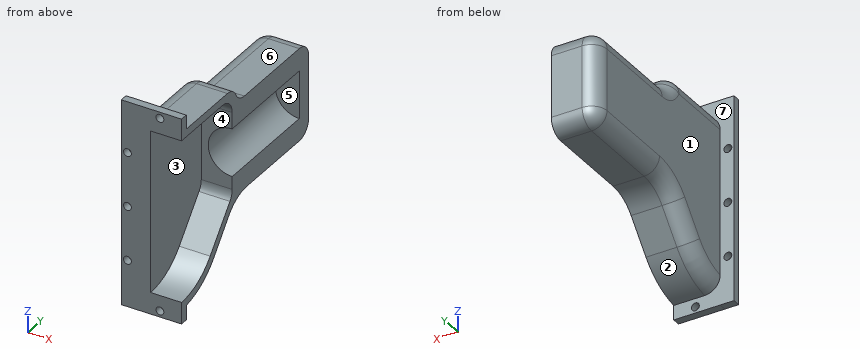
```python
from build123d import *

# Parameters (mm, degrees)
BOSS_EXTRUDE1_DEPTH   = 120
FILLET1_R             = 20
FILLET2_R             = 20
SKETCH2_W             = 18
SKETCH2_H             = 103
BOSS_EXTRUDE2_DEPTH   = 10
F_1_0MM_DOWEL_HOLE1_D = 10.2
F_1_0MM_DOWEL_HOLE2_D = 10.2
SKETCH7_R             = 31
CUT_EXTRUDE1_DEPTH    = 250
CUT_EXTRUDE2_DEPTH    = 40
BOSS_EXTRUDE3_START   = -20
BOSS_EXTRUDE3_DEPTH   = 20
SKETCH12_W            = 357.858152506
SKETCH12_H            = 320.052587915
CUT_EXTRUDE3_DEPTH    = 78


with BuildPart() as part:
    # Sketch1 → Boss-Extrude1 (new body)
    with BuildSketch(Plane(origin=(0, 0, 0), x_dir=(0, 0, -1), z_dir=(1, 0, 0))):
        with BuildLine():
            Line((0, 0), (0, 10))
            Line((0, 10), (18, 10))
            Line((18, 10), (18, 97.5))
            ThreePointArc((18, 97.5), (21.013571696, 108.05752118), (29.146125346, 115.433457659))
            ThreePointArc((29.146125346, 115.433457659), (37.278678997, 122.809394139), (40.292250693, 133.366915319))
            Line((40.292250693, 133.366915319), (40.292250693, 250))
            ThreePointArc((40.292250693, 250), (46.150115069, 264.142135624), (60.292250693, 270))
            Line((60.292250693, 270), (140.292250693, 270))
            ThreePointArc((140.292250693, 270), (154.434386317, 264.142135624), (160.292250693, 250))
            Line((160.292250693, 250), (160.292250693, 138.688740716))
            ThreePointArc((160.292250693, 138.688740716), (164.976861341, 117.557827629), (178.152870209, 100.38651856))
            Line((178.152870209, 100.38651856), (215.624604805, 68.943999881))
            ThreePointArc((215.624604805, 68.943999881), (237.098685885, 42.515288741), (247.216439033, 10))
            Line((247.216439033, 10), (266, 10))
            Line((266, 10), (266, 0))
            Line((266, 0), (147.773719933, 0))
            ThreePointArc((147.773719933, 0), (128, 23), (108.226280067, 0))
            Line((108.226280067, 0), (0, 0))
        make_face()
    extrude(amount=BOSS_EXTRUDE1_DEPTH)

    # Fillet1
    fillet1_edges = [part.edges().sort_by_distance(p)[0] for p in [
        (120, 42.515288741, -237.098685885),
        (120, 84.66525922, -196.888737507),
        (120, 117.557827629, -164.976861341),
        (120, 194.344370358, -160.292250693),
        (120, 264.142135624, -154.434386317),
        (120, 270, -100.292250693),
        (120, 264.142135624, -46.150115069),
        (120, 191.683457659, -40.292250693),
        (120, 122.809394139, -37.278678997),
        (120, 108.05752118, -21.013571696),
        (120, 53.75, -18),
    ]]
    fillet(fillet1_edges, radius=FILLET1_R)

    # Fillet2
    fillet2_edges = [part.edges().sort_by_distance(p)[0] for p in [
        (0, 53.75, -18),
        (0, 108.05752118, -21.013571696),
        (0, 122.809394139, -37.278678997),
        (0, 191.683457659, -40.292250693),
        (0, 264.142135624, -46.150115069),
        (0, 270, -100.292250693),
        (0, 264.142135624, -154.434386317),
        (0, 194.344370358, -160.292250693),
        (0, 117.557827629, -164.976861341),
        (0, 84.66525922, -196.888737507),
        (0, 42.515288741, -237.098685885),
    ]]
    fillet(fillet2_edges, radius=FILLET2_R)

    # Sketch2 → Boss-Extrude2 (add)
    with BuildSketch(Plane(origin=(0, 10, 0), x_dir=(1, 0, 0), z_dir=(0, 1, 0))):
        Polygon((-17.998263805, -0.25), (138, -0.25), (138, 93.5), (120, 93.5), (120, 0), (0, 0), (0, 265.971156308), (-17.998263805, 266), align=None)
        with Locations((129, 214.5)):
            Rectangle(SKETCH2_W, SKETCH2_H)
    extrude(amount=-BOSS_EXTRUDE2_DEPTH)

    # Ø1.0mm Dowel Hole1 (through all)
    with Locations(Plane(origin=(0, 10, 0), x_dir=(1, 0, 0), z_dir=(0, 1, 0))):
        with Locations((32.001736195, 258), (82.001736195, 258)):
            Hole(F_1_0MM_DOWEL_HOLE1_D / 2)

    # Ø1.0mm Dowel Hole2 (through all)
    with Locations(Plane(origin=(0, 10, 0), x_dir=(1, 0, 0), z_dir=(0, 1, 0))):
        with Locations((-9.998263805, 205.75), (-9.998263805, 135.75), (-9.998263805, 65.75), (32.001736195, 7.75), (82.001736195, 7.75), (130, 65.75), (130, 205.75)):
            Hole(F_1_0MM_DOWEL_HOLE2_D / 2)

    # Sketch7 → Cut-Extrude1 (cut)
    with BuildSketch(Plane.XZ):
        with Locations(Location((60.001736195, -100.29, 0), (0, 0, 270))):
            Circle(SKETCH7_R)
    extrude(amount=-CUT_EXTRUDE1_DEPTH, mode=Mode.SUBTRACT)

    # Sketch9 → Cut-Extrude2 (cut, symmetric)
    with BuildSketch(Plane(origin=(60, 0, 0), x_dir=(0, 0, -1), z_dir=(1, 0, 0))):
        with BuildLine():
            Line((28, 0), (28, 87.5))
            ThreePointArc((28, 87.5), (33.857864376, 101.642135624), (48, 107.5))
            Line((48, 107.5), (148, 107.5))
            ThreePointArc((148, 107.5), (154.928315168, 106.261621703), (160.998642822, 102.699844894))
            Line((160.998642822, 102.699844894), (209.994571286, 60.799379576))
            ThreePointArc((209.994571286, 60.799379576), (230.662114279, 33.469645181), (238, 0))
            Line((238, 0), (158, 0))
            Line((158, 0), (147.773719933, 0))
            ThreePointArc((147.773719933, 0), (128, 23), (108.226280067, 0))
            Line((108.226280067, 0), (28, 0))
        make_face()
    extrude(amount=CUT_EXTRUDE2_DEPTH, both=True, mode=Mode.SUBTRACT)

    # Sketch10 → Boss-Extrude3 (add)
    with BuildSketch(Plane(origin=(20, 0, 0), x_dir=(0, 0, -1), z_dir=(1, 0, 0)).offset(BOSS_EXTRUDE3_START)):
        with BuildLine():
            ThreePointArc((148, 3), (128, 23), (108, 3))
            Line((108, 3), (148, 3))
        make_face()
        with BuildLine():
            ThreePointArc((108, 3), (108.056650248, 1.495739163), (108.226280067, 0))
            Line((108.226280067, 0), (147.773719933, 0))
            ThreePointArc((147.773719933, 0), (147.943349752, 1.495739163), (148, 3))
            Line((148, 3), (108, 3))
        make_face()
    extrude(amount=BOSS_EXTRUDE3_DEPTH)

    # Sketch12 → Cut-Extrude3 (cut)
    with BuildSketch(Plane(origin=(138, 0, 0), x_dir=(0, 0, -1), z_dir=(1, 0, 0))):
        with Locations((133.670062861, 122.61081936)):
            Rectangle(SKETCH12_W, SKETCH12_H)
    extrude(amount=-CUT_EXTRUDE3_DEPTH, mode=Mode.SUBTRACT)


solid = part.part
```
The model under review builds one solid part; all positions refer to its coordinate system, in mm. Face numbers are marked on the shaded views. A direction names the side the tool comes from. Coordinates: 2 decimals unless noted, no trailing zeros. Order: outer loops, then holes, each group sorted by start corner. A loop starts at its lowest first (then second) coordinate and runs counter-clockwise, first axis right, second up. Notation, with made-up numbers: (66, 58) -> (79, 58) arc R37 ccw to (79, 95) -> close; hole circle Ø9 at (44, -27). An arc over 180 degrees is marked (long way). Answer in a Markdown table with one row per item. Add a question column.
Item 1: We need section A-A on z = -258. Write out the cut boundary in (x, y).
Item 2: We need section C-C on x = 46.5. Write out the cut boundary in (y, z), plus the area to 3 significant figures.
Item 3: To check wall thickness, follow probe 1 along X at (y, z) = (6, -258); probe 2 along X at (y, z) = (6.5, -135.75); probe 3 along Z at (x, y) = (45, 75.5). State the ranges of each line that lie inside material, in increasing order.
Item 4: Machinability: for the marked faces 5, 6 and 7, which of the approach directions +Z, -Z, +X, -X, +Y, -Y give a long, thin tool a straight path to every point of the face, cutting with its end or side? Answer none if there is none.
Item 5: We need section B-B on y = 232. Write out the cut boundary in (x, z).
Item 6: Clearance check with flat-ended pins moving along their axes: pin 1 (3 mm diameter, centred on y = 181.5, z = -100, fed in from -X); pin 2 (20 mm diameter, centred on x = 39.5, y = 198.5, fed in from -Z); pin 3 (6 mm diameter, centred on x = 51.5, z = -219.5, fed in from +Y). State where each tip first meets the part, or that it passes through.
Item 7: Mouldability with a two-part tool opening along Z and no side actions: class the marked faces 1, 2, 3 and 4 as +Z half, -Z half, draft (parallel to the pull), parting line (faces both ways), or undercut.
Item 8: We need section D-D on z = -65.75. Write out the cut boundary in (x, y), plus the area to 3 significant figures.
Final values:
| question | item | result |
|---|---|---|
| 1 | outline | (-18, 0) -> (26.9, 0) -> (26.9, 10) -> (-18, 10) -> close; (37.1, 0) -> (60, 0) -> (60, 10) -> (37.1, 10) -> close |
| 2 | outline | (0, -266) -> (10, -266) -> (10, -247.22) arc R90 ccw to (68.94, -215.62) -> (100.39, -178.15) arc R50 cw to (138.69, -160.29) -> (250, -160.29) arc R20 ccw to (270, -140.29) -> (270, -60.29) arc R20 ccw to (250, -40.29) -> (133.37, -40.29) arc R20 cw to (115.43, -29.15) arc R20 ccw to (97.5, -18) -> (10, -18) -> (10, 0.25) -> (0, 0.25) -> (0, -28) -> (87.5, -28) arc R20 cw to (107.5, -48) -> (107.5, -72.38) -> (250, -72.38) -> (250, -128.2) -> (107.5, -128.2) -> (107.5, -148) arc R20 cw to (102.7, -161) -> (60.8, -209.99) arc R80 cw to (0, -238) -> close |
| 2 | area | 14,600 mm2 |
| 3 | probe 1 | x = -18 to 26.9, 37.1 to 60 |
| 3 | probe 2 | x = -18 to -15.1, -4.9 to 20 |
| 3 | probe 3 | z = -207.81 to -192.8, -28 to -18 |
| 4 | face 5 | +X, -Y |
| 4 | face 6 | +Z, +X, -X, +Y |
| 4 | face 7 | -X, +Y |
| 5 | outline | (0, -140.29) arc R20 ccw to (20, -160.29) -> (60, -160.29) -> (60, -131.29) arc R31 cw to (60, -69.29) -> (60, -40.29) -> (20, -40.29) arc R20 ccw to (0, -60.29) -> close |
| 6 | pin 1 | stops at x = 0 |
| 6 | pin 2 | stops at z = -160.29 |
| 6 | pin 3 | stops at y = 68.2 |
| 7 | face 1 | draft |
| 7 | face 2 | -Z half |
| 7 | face 3 | undercut |
| 7 | face 4 | undercut |
| 8 | outline | (-18, 0) -> (-15.1, 0) -> (-15.1, 10) -> (-18, 10) -> close; (-4.9, 0) -> (20, 0) -> (20, 107.5) -> (60, 107.5) -> (60, 270) -> (20, 270) arc R20 ccw to (0, 250) -> (0, 10) -> (-4.9, 10) -> close |
| 8 | area | 11,900 mm2 |
